```python
from build123d import *

# Parameters (mm, degrees)
F0_R     = 15.25
F0_R_2   = 10.7
F1_DEPTH = 34.3
F0_R_3   = 5.85
F2_DEPTH = 39.7
F3_DEPTH = 25.4


with BuildPart() as f1:
    # F0 (on Top) → F1 (new body)
    with BuildSketch(Plane.XY):
        Circle(F0_R)
        Circle(F0_R_2, mode=Mode.SUBTRACT)
    extrude(amount=F1_DEPTH)

    # F0 (on Top) → F2 (join)
    with BuildSketch(Plane.XY):
        Circle(F0_R_2)
        Circle(F0_R_3, mode=Mode.SUBTRACT)
    extrude(amount=F2_DEPTH)

    # F0 (on Top) → F3 (join)
    with BuildSketch(Plane.XY):
        Circle(F0_R_3)
    extrude(amount=F3_DEPTH)


solid = f1.part
```
Design review of the part built by this model. Coordinates are the model's own, in mm. A direction names the side the tool comes from. Give positions to 0.01 mm unless a question says otherwise; leave off trailing zeros. Write each loop counter-clockwise with the first axis right and the second up, starting at its lowest first coordinate (ties: lowest second). Pieces come first, ordered by that corner, then holes. Notation, with made-up numbers: (-35.75, -25.5) - (-3.75, -25.5) arc R27 ccw to (-3.75, 8.5) - close; hole circle Ø2 at (43, 65). An arc over 180 degrees is marked (long way). Return JSON: item names as keys, results as strings. Group by question number.
(1) Insertion check: pin 1 (1.5 mm diameter, centred on x = 6.5, y = -12, fed in from +Z); pin 2 (5 mm diameter, centred on y = 7, z = 7, fed in from -X); pin 3 (1.5 mm diameter, centred on y = 11, z = 9, fed in from +X). Each pin has a flat end and moves straight along its axis. Give the tip position at first contact, or say it passes through.
(2) We need section A-A, the plane y = 0. Give the boundary of the cut face in (x, z).
(3) We need section B-B, the plane z = 30. Give the boundary of the cut face in (x, y), then the cut area to 3 significant figures.
(4) Mouldability with a two-part tool opening along Y and no side actions: class faces 1 (the cylindrical face through (-12.1, -9.28, 16.91)), 2 (the flat face through (-10.4, -3.2, 34.3)), 3 (the cylindrical face through (-1.27, -5.71, 32.45)) as +Y half, -Y half, draft (parallel to the pull), parting line (faces both ways), or undercut.
(5) To check wall thickness, follow probe 1 along Y at (x, z) = (0, 35); probe 2 along Y at (x, z) = (0, 32.25); probe 3 along Z at (x, y) = (11, -3.5). State the ranges of each line that lie inside material, in increasing order.
(6) Machinability: for faces 4 (the flat face through (0, 0, 25.4)), 5 (the flat face through (0, 0, 0)), which of the approach directions +Z, -Z, +X, -X, +Y, -Y give a long, thin tool a straight path to every point of the face, cutting with its end or side? Answer none if there is none.
(7) We need section D-D, the plane y = 7.5. Give the boundary of the cut face in (x, z).
Reported:
{
 "1": {"pin 1": "stops at z = 34.3", "pin 2": "stops at x = -14.57", "pin 3": "stops at x = 11.29"},
 "2": {"outline": "(-15.25, 0) - (15.25, 0) - (15.25, 34.3) - (10.7, 34.3) - (10.7, 39.7) - (5.85, 39.7) - (5.85, 25.4) - (-5.85, 25.4) - (-5.85, 39.7) - (-10.7, 39.7) - (-10.7, 34.3) - (-15.25, 34.3) - close"},
 "3": {"outline": "circle Ø30.5 at (0, 0); hole circle Ø11.7 at (0, 0)", "area": "623 mm2"},
 "4": {"face 1": "parting line", "face 2": "draft", "face 3": "undercut"},
 "5": {"probe 1": "y = -10.7 to -5.85, 5.85 to 10.7", "probe 2": "y = -15.25 to -5.85, 5.85 to 15.25", "probe 3": "z = 0 to 34.3"},
 "6": {"face 4": "+Z", "face 5": "-Z, +X, -X, +Y, -Y"},
 "7": {"outline": "(-13.28, 0) - (13.28, 0) - (13.28, 34.3) - (7.63, 34.3) - (7.63, 39.7) - (-7.63, 39.7) - (-7.63, 34.3) - (-13.28, 34.3) - close"}
}
